from build123d import *

# Parameters (mm, degrees)
BOSS_EXTRUDE1_DEPTH                          = 10
FILLET1_R                                    = 10
SHELL1_T                                     = -3
FILLET4_R                                    = 3
SKETCH2_R                                    = 9.25
BOSS_EXTRUDE2_DEPTH                          = 5
BOSS_EXTRUDE5_START                          = -3
SKETCH18_R                                   = 9.25
BOSS_EXTRUDE5_DEPTH                          = 10
SHELL2_START                                 = 3
SHELL2_OUTLINE_R                             = 6.25
SHELL2_DEPTH                                 = 7
SKETCH17_R                                   = 5
BOSS_EXTRUDE4_DEPTH                          = 10
CBORE_FOR_M5_HEX_HEAD_CAP_SCREW3_D           = 3.4
CBORE_FOR_M5_HEX_HEAD_CAP_SCREW3_CBORE_D     = 6.5
CBORE_FOR_M5_HEX_HEAD_CAP_SCREW3_CBORE_DEPTH = 3


# Read off the part's stored shape, not the designer's step: Shell2
with BuildPart() as part:
    # Sketch1 → Boss-Extrude1 (new body)
    with BuildSketch(Plane.XY):
        with BuildLine():
            Line((17.67766953, -17.67766953), (98.994949366, 63.639610307))
            Line((98.994949366, 63.639610307), (98.994949366, 153.051453663))
            ThreePointArc((98.994949366, 153.051453663), (73.994949366, 178.051453663), (48.994949366, 153.051453663))
            Line((48.994949366, 153.051453663), (48.994949366, 84.350288425))
            Line((48.994949366, 84.350288425), (-17.67766953, 17.67766953))
            ThreePointArc((-17.67766953, 17.67766953), (-17.67766953, -17.67766953), (17.67766953, -17.67766953))
        make_face()
    extrude(amount=BOSS_EXTRUDE1_DEPTH)

    # Fillet1
    fillet1_edges = [part.edges().sort_by_distance(p)[0] for p in [
        (48.994949366, 84.350288425, 5),
        (98.994949366, 63.639610307, 5),
    ]]
    fillet(fillet1_edges, radius=FILLET1_R)

    # Shell1
    shell1_openings = [part.faces().sort_by_distance(p)[0] for p in [
        (50.162308395, 71.072674162, 10),
    ]]
    offset(amount=SHELL1_T, openings=shell1_openings, kind=Kind.INTERSECTION)

    # Fillet4
    fillet4_edges = [part.edges().sort_by_distance(p)[0] for p in [
        (98.994949366, 110.416599797, 0),
        (14.194173824, 49.549512883, 0),
        (98.233744691, 63.954911607, 0),
        (48.233744691, 84.665589726, 0),
        (48.994949366, 120.771938856, 0),
        (73.994949366, 178.051453663, 0),
        (56.871843354, 21.516504294, 0),
        (-17.67766953, -17.67766953, 0),
    ]]
    fillet(fillet4_edges, radius=FILLET4_R)

    # Sketch2 → Boss-Extrude2 (add)
    with BuildSketch(Plane.XY.offset(3)):
        Circle(SKETCH2_R)
    extrude(amount=BOSS_EXTRUDE2_DEPTH)

    # Sketch18 → Boss-Extrude5 (add)
    with BuildSketch(Plane.XY.offset(3).offset(BOSS_EXTRUDE5_START)):
        with Locations((73.994949366, 153.051453663)):
            Circle(SKETCH18_R)
    extrude(amount=BOSS_EXTRUDE5_DEPTH)

    # Shell2 outline → Shell2 (cut)
    with BuildSketch(Plane.XY.offset(SHELL2_START)):
        with Locations((73.994949366, 153.051453663)):
            Circle(SHELL2_OUTLINE_R)
        Circle(SHELL2_OUTLINE_R)
    extrude(amount=SHELL2_DEPTH, mode=Mode.SUBTRACT)

    # Sketch17 → Boss-Extrude4 (add)
    with BuildSketch(Plane.XY):
        with Locations((40.533008589, 58.210678119)):
            Circle(SKETCH17_R)
        with Locations((61.494949366, 108.817279836)):
            Circle(SKETCH17_R)
        with Locations((86.494949366, 108.817279836)):
            Circle(SKETCH17_R)
        with Locations((58.210678119, 40.533008589)):
            Circle(SKETCH17_R)
    extrude(amount=BOSS_EXTRUDE4_DEPTH)

    # CBORE for M5 Hex Head Cap Screw3 (through all)
    with Locations(Plane(origin=(0, 0, 0), x_dir=(-1, 0, 0), z_dir=(0, 0, -1))):
        with Locations((-86.494949366, 108.817279836), (-61.494949366, 108.817279836), (-58.210678119, 40.533008589), (-40.533008589, 58.210678119)):
            CounterBoreHole(CBORE_FOR_M5_HEX_HEAD_CAP_SCREW3_D / 2, CBORE_FOR_M5_HEX_HEAD_CAP_SCREW3_CBORE_D / 2, CBORE_FOR_M5_HEX_HEAD_CAP_SCREW3_CBORE_DEPTH)


solid = part.part
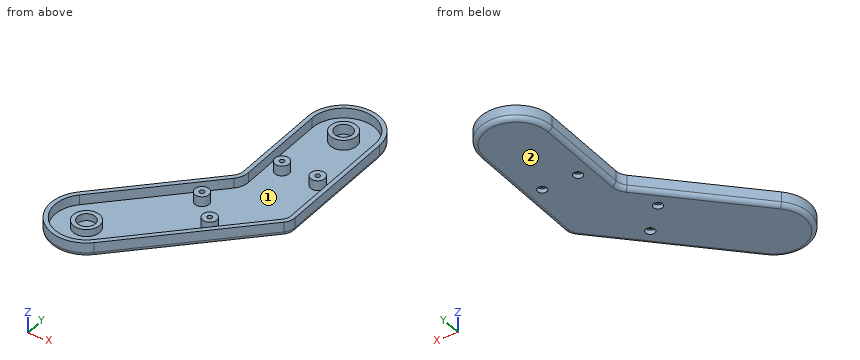
The listing builds one solid part. Answer for the finished solid, in the listing's coordinates (mm). Face numbers are marked on the shaded views. Give positions to 0.01 mm unless a question says otherwise; leave off trailing zeros. Write each loop counter-clockwise with the first axis right and the second up, starting at its lowest first coordinate (ties: lowest second). Pieces come first, ordered by that corner, then holes.
Item 1: Section A-A, the plane z = 5.5 is taken. Count the separate pieces of the cut face and the enclosed holes in it, plus the area to 3 significant figures.
Item 2: Section B-B, the plane y = 133 is taken. Write down the section's boundary in (x, z).
Item 3: Determine the mould class of the marked faces 1 and 2 for opening direction X: released by +X, released by -X, zero draft, split by the parting line, or undercut.
Item 4: Flat-ended cylindrical pins translate along their axes: P1, Ø8.5, axis at x = 61.49, y = 108.82, coming from the -Z side; P2, Ø6, axis at x = 3, y = -1, coming from the +Z side; P3, Ø2, axis at x = 61.49, y = 108.82, coming from the -Z side; P4, Ø5.5, axis at y = 106, z = 6.5, coming from the -X side. Find the tip coordinate at first contact, or state that the pin passes through.
Item 5: Find the intervals of material crossed by line 1 along X through (y, z) = (137, 9.75); line 2 along Y through (x, z) = (86, 6.75); line 3 along Y through (x, z) = (0, 6.75), in increasing order.
Completed:
1. separate pieces: 7
1. enclosed holes: 7
1. area: 2,110 mm2
2. outline: (48.99, 3) arc R3 ccw to (51.99, 0) - (95.99, 0) arc R3 ccw to (98.99, 3) - (98.99, 10) - (95.99, 10) - (95.99, 3) - (51.99, 3) - (51.99, 10) - (48.99, 10) - close
3. face 1: undercut
3. face 2: zero draft
4. P1: stops at z = 0
4. P2: stops at z = 3
4. P3: passes through
4. P4: stops at x = 48.99
5. line 1: x = 48.99 to 51.99, 95.99 to 98.99
5. line 2: y = 50.64 to 54.89, 103.84 to 107.19, 110.44 to 113.79, 171.49 to 174.98
5. line 3: y = -25 to -22, -9.25 to -6.25, 6.25 to 9.25, 31.11 to 35.36
